```python
from build123d import *

# Parameters (mm, degrees)
PAD003_DEPTH      = 4
SKETCH002_R       = 12
PAD_DEPTH         = 9
SKETCH003_R       = 5
PAD004_DEPTH      = 13
SKETCH001_R       = 4
SKETCH001_R_2     = 2.5
POCKET_DEPTH      = 0.001
POCKET_DEPTH_BACK = -13.001


with BuildPart() as part:
    # Sketch004 → Pad003 (new body)
    with BuildSketch(Plane.XY):
        with BuildLine():
            ThreePointArc((-21.23684, 4.47175), (-24, 0), (-21.23684, -4.47175))
            Line((-21.23684, -4.47175), (-6.039475, -12.073721))
            ThreePointArc((-6.039475, -12.073721), (0, -13.5), (6.039474, -12.073722))
            Line((6.039474, -12.073722), (21.236823, -4.471758))
            ThreePointArc((21.236823, -4.471758), (24, 0), (21.236823, 4.471758))
            Line((6.039474, 12.073722), (21.236823, 4.471758))
            ThreePointArc((6.039474, 12.073722), (0, 13.5), (-6.039475, 12.073721))
            Line((-21.23684, 4.47175), (-6.039475, 12.073721))
        make_face()
    extrude(amount=PAD003_DEPTH)

    # Sketch002 → Pad (join)
    with BuildSketch(Plane.XY):
        Circle(SKETCH002_R)
    extrude(amount=PAD_DEPTH)

    # Sketch003 → Pad004 (join)
    with BuildSketch(Plane.XY):
        Circle(SKETCH003_R)
    extrude(amount=PAD004_DEPTH)

    # Sketch001 → Pocket (cut, two sides)
    with BuildSketch(Plane.XY) as pocket_sk:
        Circle(SKETCH001_R)
        with Locations((18.25, 0)):
            Circle(SKETCH001_R_2)
        with Locations((-18.25, 0)):
            Circle(SKETCH001_R_2)
    extrude(amount=-POCKET_DEPTH, mode=Mode.SUBTRACT)
    extrude(pocket_sk.sketch, amount=-POCKET_DEPTH_BACK, mode=Mode.SUBTRACT)


solid = part.part
```
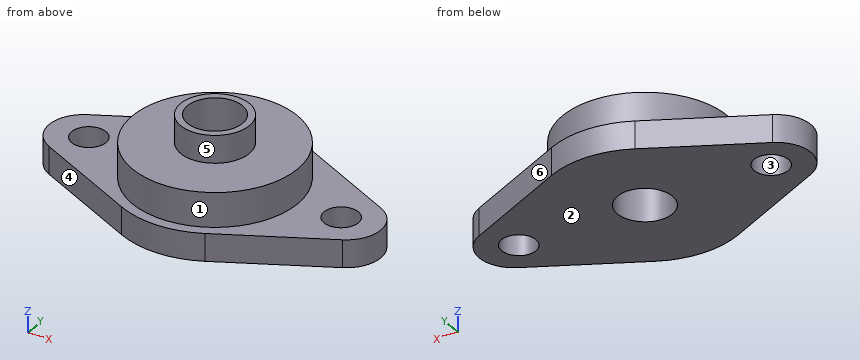
Input: part model. Units: mm. Frame: model coordinates. Face numbers are marked on the shaded views. A direction names the side the tool comes from. Coordinates: 2 decimals unless noted, no trailing zeros. Write each loop counter-clockwise with the first axis right and the second up, starting at its lowest first coordinate (ties: lowest second). Pieces come first, ordered by that corner, then holes. Notation, with made-up numbers: (66.25, 79) - (83.25, 79) arc R22 cw to (83.25, 103) - close; hole circle Ø2 at (87.5, 1.25). An arc over 180 degrees is marked (long way). Put each result on its own line as item: value. Start each with the question number.
1) Cut plane D-D (x = -18.25). Return the cut outline in (y, z), plus the area to 3 significant figures.
2) Contact query for flat-ended pins moving along their axis: pin 1 (1.5 mm diameter, centred on x = 1, y = -8, fed in from +Z); pin 2 (6 mm diameter, centred on y = 7.5, z = 4.5, fed in from -X); pin 3 (5 mm diameter, centred on x = -8, z = 8, fed in from -Y); pin 4 (1 mm diameter, centred on y = 7.5, z = 10, fed in from +X). Output: stop coordinate, or through.
3) Cut plane A-A (x = 0). Return the cut outline in (y, z).
4) Cut plane B-B (y = 0). Return the cut outline in (x, z), plus the area to 3 significant figures.
5) Mould query, pull axis Y, two halves, no side actions, for the marked faces 3, 4, 5 and 6. Classes: pulls with the +Y half, pulls with the -Y half, needs draft (parallel to the pull), parting line crosses it, or undercut.
6) Ray query, L1, parallel to Y at x = 0, z = 7.25; L2, parallel to X at y = 0, z = 9.5. Return the intervals inside material, ascending.
7) Cut plane C-C (z = 5.5). Return the cut outline in (x, y).
8) Reachability of the marked faces 1 and 2 from +Z, -Z, +X, -X, +Y, -Y: full face, straight path, thin tool, end or side. Return the list, or none.
Resolved:
1. outline: (-5.97, 0) - (-2.5, 0) - (-2.5, 4) - (-5.97, 4) - close; (2.5, 0) - (5.97, 0) - (5.97, 4) - (2.5, 4) - close
1. area: 27.7 mm2
2. pin 1: stops at z = 9
2. pin 2: stops at x = -21.1
2. pin 3: stops at y = -10.67
2. pin 4: passes through
3. outline: (-13.5, 0) - (-4, 0) - (-4, 13) - (-5, 13) - (-5, 9) - (-12, 9) - (-12, 4) - (-13.5, 4) - close; (4, 0) - (13.5, 0) - (13.5, 4) - (12, 4) - (12, 9) - (5, 9) - (5, 13) - (4, 13) - close
4. outline: (-24, 0) - (-20.75, 0) - (-20.75, 4) - (-24, 4) - close; (-15.75, 0) - (-4, 0) - (-4, 13) - (-5, 13) - (-5, 9) - (-12, 9) - (-12, 4) - (-15.75, 4) - close; (4, 0) - (15.75, 0) - (15.75, 4) - (12, 4) - (12, 9) - (5, 9) - (5, 13) - (4, 13) - close; (20.75, 0) - (24, 0) - (24, 4) - (20.75, 4) - close
4. area: 208 mm2
5. face 3: undercut
5. face 4: pulls with the -Y half
5. face 5: parting line crosses it
5. face 6: pulls with the +Y half
6. L1: y = -12 to -4, 4 to 12
6. L2: x = -5 to -4, 4 to 5
7. outline: circle Ø24 at (0, 0); hole circle Ø8 at (0, 0)
8. face 1: +Z
8. face 2: -Z, +X, -X, +Y, -Y
